Input: part model. Units: mm. Frame: model coordinates. A direction names the side the tool comes from. Coordinates: 2 decimals unless noted, no trailing zeros. Write each loop counter-clockwise with the first axis right and the second up, starting at its lowest first coordinate (ties: lowest second). Pieces come first, ordered by that corner, then holes.
from build123d import *

# Parameters (mm, degrees)
F0_R     = 37
F1_DEPTH = 4.5
F3_DEPTH = 3.5
F5_DEPTH = 15
F6_R     = 1.65
F7_DEPTH = 4.501
F9_DEPTH = 3


with BuildPart() as f1:
    # F0 (on Top) → F1 (new body)
    with BuildSketch(Plane.XY):
        Circle(F0_R)
    extrude(amount=F1_DEPTH)

    # F2 (on face) → F3 (cut)
    with BuildSketch(Plane(origin=(0, 0, 0), x_dir=(1, 0, 0), z_dir=(0, 0, -1))):
        with BuildLine():
            ThreePointArc((3.479853, -0.375), (3.49496, -0.18777), (3.5, 0))
            ThreePointArc((3.5, 0), (3.49496, 0.18777), (3.479853, 0.375))
            ThreePointArc((3.479853, 0.375), (2.338536, 2.604083), (0, 3.5))
            ThreePointArc((0, 3.5), (-2.338536, 2.604083), (-3.479853, 0.375))
            ThreePointArc((-3.479853, 0.375), (-3.5, 0), (-3.479853, -0.375))
            ThreePointArc((-3.479853, -0.375), (0, -3.5), (3.479853, -0.375))
        make_face()
        with BuildLine():
            ThreePointArc((0, 3.5), (2.338536, 2.604083), (3.479853, 0.375))
            Line((3.479853, 0.375), (1.988487, 14.214286))
            ThreePointArc((1.988487, 14.214286), (1.99712, 14.107297), (2, 14))
            ThreePointArc((2, 14), (1.414214, 12.585786), (0, 12))
            Line((0, 12), (0, 3.5))
        make_face()
        with BuildLine():
            Line((1.988487, -14.214286), (3.479853, -0.375))
            ThreePointArc((3.479853, -0.375), (0, -3.5), (-3.479853, -0.375))
            Line((-3.479853, -0.375), (-1.988487, -14.214286))
            ThreePointArc((-1.988487, -14.214286), (-0.107297, -12.00288), (2, -14))
            ThreePointArc((2, -14), (1.99712, -14.107297), (1.988487, -14.214286))
        make_face()
        with BuildLine():
            ThreePointArc((-3.479853, 0.375), (-2.338536, 2.604083), (0, 3.5))
            Line((0, 3.5), (0, 12))
            ThreePointArc((0, 12), (-1.488048, 12.663694), (-1.988487, 14.214286))
            Line((-1.988487, 14.214286), (-3.479853, 0.375))
        make_face()
        with BuildLine():
            ThreePointArc((2, 14), (1.99712, 14.107297), (1.988487, 14.214286))
            ThreePointArc((1.988487, 14.214286), (0, 16), (-1.988487, 14.214286))
            ThreePointArc((-1.988487, 14.214286), (-1.488048, 12.663694), (0, 12))
            ThreePointArc((0, 12), (1.414214, 12.585786), (2, 14))
        make_face()
        with BuildLine():
            ThreePointArc((-1.988487, -14.214286), (0, -16), (1.988487, -14.214286))
            ThreePointArc((1.988487, -14.214286), (1.99712, -14.107297), (2, -14))
            ThreePointArc((2, -14), (-0.107297, -12.00288), (-1.988487, -14.214286))
        make_face()
    extrude(amount=-F3_DEPTH, mode=Mode.SUBTRACT)

    # F4 (on Right) → F5 (join, symmetric)
    with BuildSketch(Plane.YZ):
        with BuildLine():
            ThreePointArc((-20, 8.5), (-22.828427, 7.328427), (-24, 4.5))
            Line((-24, 4.5), (-20, 4.5))
            Line((-20, 4.5), (-20, 8.5))
        make_face()
        with BuildLine():
            Line((20, 8.5), (20, 4.5))
            Line((20, 4.5), (24, 4.5))
            ThreePointArc((24, 4.5), (22.828427, 7.328427), (20, 8.5))
        make_face()
    extrude(amount=F5_DEPTH, both=True)

    # F6 (on face) → F7 (cut, through all)
    with BuildSketch(Plane.XY.offset(4.5)):
        with Locations((-24, 0)):
            Circle(F6_R)
        with Locations((24, 0)):
            Circle(F6_R)
    extrude(amount=-F7_DEPTH, mode=Mode.SUBTRACT)

    # F8 (on face) → F9 (cut)
    with BuildSketch(Plane(origin=(0, 0, 0), x_dir=(1, 0, 0), z_dir=(0, 0, -1))):
        Polygon((22.412287, 2.75), (20.824574, 0), (22.412287, -2.75), (25.587713, -2.75), (27.175426, 0), (25.587713, 2.75), align=None)
        Polygon((-22.412287, -2.75), (-20.824574, 0), (-22.412287, 2.75), (-25.587713, 2.75), (-27.175426, 0), (-25.587713, -2.75), align=None)
    extrude(amount=-F9_DEPTH, mode=Mode.SUBTRACT)


solid = f1.part
Item 1: Pin query (flat end, axial travel): pin 1 Ø1.2 at (y, z) = (-22, 5.5) entering from -X; pin 2 Ø3.5 at (x, z) = (24.5, 2) entering from -Y; pin 3 Ø0.9 at (x, z) = (24, 1) entering from +Y. Return the tip coordinate at first contact, or that it passes through.
Item 2: Material intervals for line 1 (Z direction, x = 19, y = -1.5); line 2 (Z direction, x = -25, y = -2.5); line 3 (Y direction, x = 6, z = 7), sorted ascending.
Item 3: Section query D-D, the plane y = -7.5. Return loops of the section in (x, z).
Item 4: Section query B-B, the plane x = 0. Return loops of the section in (y, z).
Item 5: Section query A-A, the plane x = 24. Return loops of the section in (y, z).
Item 6: Section query C-C, the plane z = 7. Return loops of the section in (x, y).
Item 7: Access query for faces 1 (the face through (0.21, 22.859, 7.297)), 2 (the face through (15, 22, 6)), 3 (the face through (0, 0, 3.5)), 4 (the face through (-15, 22, 6)). Directions: +Z, -Z, +X, -X, +Y, -Y. A direction counts if a zero-diameter tool reaches every point of the face in a straight line with its end or side. Return the directions, or none.
Item 8: Pull-direction query (X, two-part tool) for faces 5 (the face through (-15, -22, 6)), 6 (the face through (15, -22, 6)), 7 (the face through (22.35, 0.07, 3.76)), 8 (the face through (0, -20, 6)); classes: released by +X, released by -X, zero draft, split by the parting line, or undercut.
The answers:
1. pin 1: stops at x = -15
1. pin 2: stops at y = -29.18
1. pin 3: stops at y = 28.54
2. line 1: z = 0 to 4.5
2. line 2: z = 3 to 4.5
2. line 3: y = -23.12 to -20, 20 to 23.12
3. outline: (-36.23, 0) - (-2.71, 0) - (-2.71, 3.5) - (2.71, 3.5) - (2.71, 0) - (36.23, 0) - (36.23, 4.5) - (-36.23, 4.5) - close
4. outline: (-37, 0) - (-16, 0) - (-16, 3.5) - (16, 3.5) - (16, 0) - (37, 0) - (37, 4.5) - (24, 4.5) arc R4 ccw to (20, 8.5) - (20, 4.5) - (-20, 4.5) - (-20, 8.5) arc R4 ccw to (-24, 4.5) - (-37, 4.5) - close
5. outline: (-28.16, 0) - (-2.75, 0) - (-2.75, 3) - (-1.65, 3) - (-1.65, 4.5) - (-28.16, 4.5) - close; (1.65, 3) - (2.75, 3) - (2.75, 0) - (28.16, 0) - (28.16, 4.5) - (1.65, 4.5) - close
6. outline: (-15, -23.12) - (15, -23.12) - (15, -20) - (-15, -20) - close; (-15, 20) - (15, 20) - (15, 23.12) - (-15, 23.12) - close
7. face 1: +Z, +X, -X, +Y
7. face 2: +Z, +X, +Y, -Y
7. face 3: -Z
7. face 4: +Z, -X, +Y, -Y
8. face 5: released by -X
8. face 6: released by +X
8. face 7: undercut
8. face 8: zero draft
